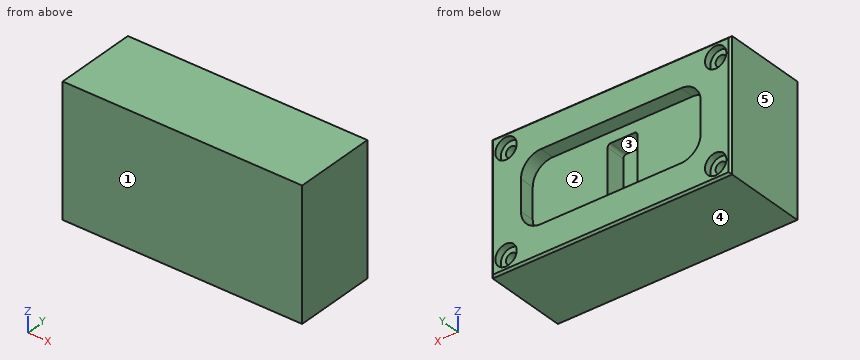
```python
from build123d import *

# Parameters (mm, degrees)
SKETCH3_W                                = 240.765342714
SKETCH3_H                                = 130.947670476
BOSS_EXTRUDE2_DEPTH                      = 85
SKETCH4_W                                = 180.765342714
SKETCH4_H                                = 70.947670476
CUT_EXTRUDE1_DEPTH                       = 15
CBORE_FOR_M10_HEX_HEAD_BOLT1_D           = 11
CBORE_FOR_M10_HEX_HEAD_BOLT1_DEPTH       = 20
CBORE_FOR_M10_HEX_HEAD_BOLT1_CBORE_D     = 21.48
CBORE_FOR_M10_HEX_HEAD_BOLT1_CBORE_DEPTH = 6.85
CBORE_FOR_M10_HEX_HEAD_BOLT1_TIP         = 3.304733405
FILLET1_R                                = 20
CHAMFER1_SIZE                            = 2
CUT_EXTRUDE2_DEPTH                       = 20


with BuildPart() as part:
    # Sketch3 → Boss-Extrude2 (new body)
    with BuildSketch(Plane(origin=(0, 0, 0), x_dir=(1, 0, 0), z_dir=(0, 1, 0))):
        Rectangle(SKETCH3_W, SKETCH3_H)
    extrude(amount=BOSS_EXTRUDE2_DEPTH)

    # Sketch4 → Cut-Extrude1 (cut)
    with BuildSketch(Plane(origin=(0, 85, 0), x_dir=(1, 0, 0), z_dir=(0, 1, 0))):
        Rectangle(SKETCH4_W, SKETCH4_H)
    extrude(amount=-CUT_EXTRUDE1_DEPTH, mode=Mode.SUBTRACT)

    # CBORE for M10 Hex Head Bolt1
    with Locations(Plane(origin=(-105.382671357, 85, -50.473835238), x_dir=(0, 0, 1), z_dir=(0, 1, 0))):
        with Locations((0, 0), (100.947670476, 0), (0, 210.765342714), (100.947670476, 210.765342714)):
            CounterBoreHole(CBORE_FOR_M10_HEX_HEAD_BOLT1_D / 2, CBORE_FOR_M10_HEX_HEAD_BOLT1_CBORE_D / 2, CBORE_FOR_M10_HEX_HEAD_BOLT1_CBORE_DEPTH, depth=CBORE_FOR_M10_HEX_HEAD_BOLT1_DEPTH)
            with Locations((0, 0, -(CBORE_FOR_M10_HEX_HEAD_BOLT1_DEPTH + CBORE_FOR_M10_HEX_HEAD_BOLT1_TIP / 2))):  # 118° drill point
                Cone(0, CBORE_FOR_M10_HEX_HEAD_BOLT1_D / 2, CBORE_FOR_M10_HEX_HEAD_BOLT1_TIP, mode=Mode.SUBTRACT)

    # Fillet1
    fillet1_edges = [part.edges().sort_by_distance(p)[0] for p in [
        (90.382671357, 77.5, 35.473835238),
        (-90.382671357, 77.5, 35.473835238),
        (-90.382671357, 77.5, -35.473835238),
        (90.382671357, 77.5, -35.473835238),
    ]]
    fillet(fillet1_edges, radius=FILLET1_R)

    # Chamfer1
    chamfer1_edges = [part.edges().sort_by_distance(p)[0] for p in [
        (-120.382671357, 85, 0),
        (0, 85, 65.473835238),
        (120.382671357, 85, 0),
        (0, 85, -65.473835238),
    ]]
    chamfer(chamfer1_edges, length=CHAMFER1_SIZE)

    # Sketch7 → Cut-Extrude2 (cut)
    with BuildSketch(Plane(origin=(0, 70, 0), x_dir=(1, 0, 0), z_dir=(0, 1, 0))):
        with BuildLine():
            Line((-12, -25), (12, -25))
            ThreePointArc((12, -25), (14.121320344, -24.121320344), (15, -22))
            Line((15, -22), (15, 22))
            ThreePointArc((15, 22), (14.121320344, 24.121320344), (12, 25))
            Line((12, 25), (-12, 25))
            ThreePointArc((-12, 25), (-14.121320344, 24.121320344), (-15, 22))
            Line((-15, 22), (-15, -22))
            ThreePointArc((-15, -22), (-14.121320344, -24.121320344), (-12, -25))
        make_face()
    extrude(amount=-CUT_EXTRUDE2_DEPTH, mode=Mode.SUBTRACT)


solid = part.part
```
Can you work these out from the model? Positions are in its coordinate system, mm. Face numbers are marked on the shaded views. A direction names the side the tool comes from. Round coordinates to 2 decimals unless told otherwise and drop trailing zeros. Loops run counter-clockwise (first coordinate to the right, second up) from the corner with the lowest first, then second, coordinate; pieces in that order, holes last.
Item 1: Suppose I cut it at C-C, the plane z = 31.5. Write out the boundary of the cut face in (x, y), then the cut area to 3 significant figures.
Item 2: Will these pins go through, and if not, where does the flat tip stop? pin 1 Ø9 at (x, z) = (-105.38, -50.47) entering from +Y; pin 2 Ø6.5 at (x, z) = (109.5, -53.5) entering from +Y.
Item 3: Suppose I cut it at A-A, the plane y = 55.5. Write out the boundary of the cut face in (x, z).
Item 4: Suppose I cut it at B-B, the plane x = -56.5. Write out the boundary of the cut face in (y, z), then the cut area to 3 significant figures.
Item 5: Suppose I cut it at D-D, the plane z = -2. Write out the boundary of the cut face in (x, y).
Item 6: Please list where these lines run through material, in increasing order: L1, parallel to X at y = 55, z = 6; L2, parallel to Z at x = -53, y = 72; L3, parallel to X at y = 73, z = 47.
Item 7: Which directions (+Z, -Z, +X, -X, +Y, -Y) give clear straight access to the entire face, cutting with the end or side of a thin tool? Please do the marked faces 1 and 2.
Item 8: If we mould it in two halves opening along X, with no side actions, what happens to the marked faces 3, 4 and 5? For each: +X half, -X half, draft (parallel to the pull), parting line (faces both ways), or undercut.
Reported:
1. outline: (-120.38, 0) - (120.38, 0) - (120.38, 83) - (118.38, 85) - (82.35, 85) - (82.35, 70) - (-82.35, 70) - (-82.35, 85) - (-118.38, 85) - (-120.38, 83) - close
1. area: 18,000 mm2
2. pin 1: stops at y = 64.4
2. pin 2: stops at y = 78.15
3. outline: (-120.38, -65.47) - (120.38, -65.47) - (120.38, 65.47) - (-120.38, 65.47) - close; hole (-15, -22) arc R3 ccw to (-12, -25) - (12, -25) arc R3 ccw to (15, -22) - (15, 22) arc R3 ccw to (12, 25) - (-12, 25) arc R3 ccw to (-15, 22) - close
4. outline: (0, -65.47) - (83, -65.47) - (85, -63.47) - (85, -35.47) - (70, -35.47) - (70, 35.47) - (85, 35.47) - (85, 63.47) - (83, 65.47) - (0, 65.47) - close
4. area: 10,100 mm2
5. outline: (-120.38, 0) - (120.38, 0) - (120.38, 83) - (118.38, 85) - (90.38, 85) - (90.38, 70) - (15, 70) - (15, 50) - (-15, 50) - (-15, 70) - (-90.38, 70) - (-90.38, 85) - (-118.38, 85) - (-120.38, 83) - close
6. L1: x = -120.38 to -15, 15 to 120.38
6. L2: z = -65.47 to -35.47, 35.47 to 65.47
6. L3: x = -120.38 to -109.65, -101.12 to 101.12, 109.65 to 120.38
7. face 1: +Z, -Z, +X, -X, -Y
7. face 2: +Y
8. face 3: undercut
8. face 4: draft
8. face 5: -X half
